```python
from build123d import *

# Parameters (mm, degrees)
SKETCH1_R           = 26
SKETCH1_R_2         = 9
BOSS_EXTRUDE1_DEPTH = 2


with BuildPart() as part:
    # Sketch1 → Boss-Extrude1 (new body)
    with BuildSketch(Plane(origin=(0, 0, 0), x_dir=(1, 0, 0), z_dir=(0, 1, 0))):
        with Locations(Location((-0.344405321, 0.81125846, 0), (0, 0, 270))):
            Circle(SKETCH1_R)
        with Locations(Location((12.557190609, 0.81125846, 0), (0, 0, 270))):
            Circle(SKETCH1_R_2, mode=Mode.SUBTRACT)
        with Locations(Location((-13.442809391, 0.81125846, 0), (0, 0, 270))):
            Circle(SKETCH1_R_2, mode=Mode.SUBTRACT)
        with BuildLine():
            Line((-4.479671933, 10.31125846), (3.371060839, 10.31125846))
            ThreePointArc((3.371060839, 10.31125846), (5.371060839, 8.31125846), (3.371060839, 6.31125846))
            Line((3.371060839, 6.31125846), (-4.479671933, 6.31125846))
            ThreePointArc((-4.479671933, 6.31125846), (-6.479671933, 8.31125846), (-4.479671933, 10.31125846))
        make_face(mode=Mode.SUBTRACT)
    extrude(amount=BOSS_EXTRUDE1_DEPTH)


solid = part.part
```
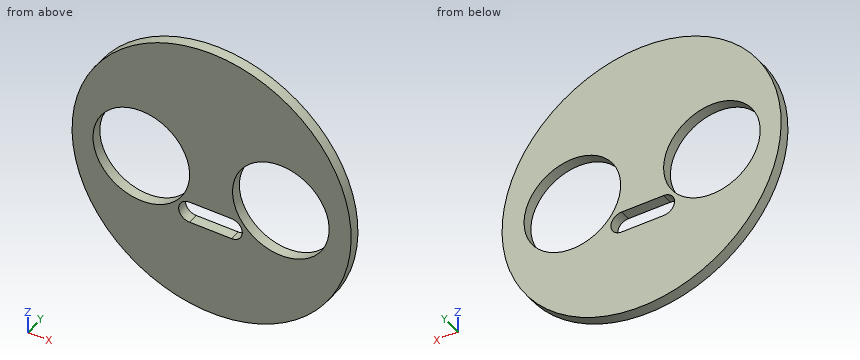
Here's how the part is built. I have some questions about the finished solid (model axes, mm). Coordinates: 2 decimals unless noted, no trailing zeros. Loops run counter-clockwise (first coordinate to the right, second up) from the corner with the lowest first, then second, coordinate; pieces in that order, holes last. Notation, with made-up numbers: (73, 73.25) -> (82, 73.25) arc R29 cw to (82, 104.25) -> close; hole circle Ø7 at (82, 9). An arc over 180 degrees is marked (long way). Return JSON: item names as keys, results as strings.
1) If we section it at D-D, the plane x = -3.5: Write out the boundary of the cut face in (y, z), then the cut area to 3 significant figures.
Results below:
{"outline": "(0, -26.62) -> (2, -26.62) -> (2, -10.31) -> (0, -10.31) -> close; (0, -6.31) -> (2, -6.31) -> (2, 25) -> (0, 25) -> close", "area": "95.2 mm²"}
2) If we section it at A-A, the plane x = 2: Write out the boundary of the cut face in (y, z).
Results below:
{"outline": "(0, -26.71) -> (2, -26.71) -> (2, -10.31) -> (0, -10.31) -> close; (0, -6.31) -> (2, -6.31) -> (2, 25.08) -> (0, 25.08) -> close"}
3) I need wall thicknesses on line 1 (X direction, y = 0.3, z = -2); line 2 (X direction, y = 1, z = -3.5) (3 decimals); line 3 (X direction, y = 1.85, z = -6.5). Which ranges of each line are inside material? Lowest first, please. Write a range as from..to.
Results below:
{"line 1": "-26.32..-22.36, -4.52..3.64, 21.48..25.63", "line 2": "-26.205..-22.032, -4.854..3.968, 21.146..25.516", "line 3": "-25.71..-20.42, -6.47..-5.33, 4.22..5.58, 19.53..25.03"}
4) Will these pins go through, and if not, where does the flat tip stop? pin 1 (11 mm diameter, centred on x = -13.44, z = -0.81, fed in from +Y); pin 2 (1 mm diameter, centred on x = -6, y = 1.5, fed in from +Z).
Results below:
{"pin 1": "through", "pin 2": "z = 24.67"}
5) If we section it at B-B, the plane y = 1.6: Write out the boundary of the cut face in (x, z).
Results below:
{"outline": "circle Ø52 at (-0.34, -0.81); hole circle Ø18 at (-13.44, -0.81); hole (-4.48, -10.31) -> (3.37, -10.31) arc R2 ccw to (3.37, -6.31) -> (-4.48, -6.31) arc R2 ccw to start; hole circle Ø18 at (12.56, -0.81)"}
6) If we section it at C-C, the plane z = -1.5: Write out the boundary of the cut face in (x, y).
Results below:
{"outline": "(-26.34, 0) -> (-22.42, 0) -> (-22.42, 2) -> (-26.34, 2) -> close; (-4.47, 0) -> (3.58, 0) -> (3.58, 2) -> (-4.47, 2) -> close; (21.53, 0) -> (25.65, 0) -> (25.65, 2) -> (21.53, 2) -> close"}
